from build123d import *

# Parameters (mm, degrees)
SKETCH1_W           = 60
SKETCH1_H           = 60
BOSS_EXTRUDE1_DEPTH = 1.2
FILLET1_R           = 4
SKETCH3_W           = 6.8
SKETCH3_H           = 20
BOSS_EXTRUDE3_DEPTH = 10
FILLET2_R           = 4
CUT_EXTRUDE1_DEPTH  = 100
CUT_EXTRUDE2_DEPTH  = 44.588989435
BOSS_EXTRUDE4_START = 10
BOSS_EXTRUDE4_DEPTH = 10
CUT_EXTRUDE4_REACH  = 55.014
SKETCH6_R           = 1.6
CUT_EXTRUDE5_REACH  = 62.463
SKETCH7_R           = 1.6
CUT_EXTRUDE6_REACH  = 62.463
SKETCH8_R           = 1.6
CUT_EXTRUDE7_REACH  = 62.463
SKETCH9_R           = 1.6
CUT_EXTRUDE8_REACH  = 62.463
SKETCH10_R          = 1.6


with BuildPart() as part:
    # Sketch1 → Boss-Extrude1 (new body)
    with BuildSketch(Plane(origin=(0, 0, 0), x_dir=(1, 0, 0), z_dir=(0, 1, 0))):
        Rectangle(SKETCH1_W, SKETCH1_H)
    extrude(amount=BOSS_EXTRUDE1_DEPTH)

    # Fillet1
    fillet1_edges = [part.edges().sort_by_distance(p)[0] for p in [
        (30, 0.6, 30),
        (-30, 0.6, 30),
        (-30, 0.6, -30),
        (30, 0.6, -30),
    ]]
    fillet(fillet1_edges, radius=FILLET1_R)

    # Sketch3 → Boss-Extrude3 (add)
    with BuildSketch(Plane(origin=(0, 1.2, 0), x_dir=(1, 0, 0), z_dir=(0, 1, 0))):
        with Locations((-25, 0)):
            Rectangle(SKETCH3_W, SKETCH3_H)
        with Locations((25, 0)):
            Rectangle(SKETCH3_W, SKETCH3_H)
    extrude(amount=BOSS_EXTRUDE3_DEPTH)

    # Fillet2
    fillet2_edges = [part.edges().sort_by_distance(p)[0] for p in [
        (-25, 11.2, -10),
        (-25, 11.2, 10),
        (25, 11.2, 10),
        (25, 11.2, -10),
    ]]
    fillet(fillet2_edges, radius=FILLET2_R)

    # Sketch4 → Cut-Extrude1 (cut)
    with BuildSketch(Plane.ZY.offset(28.4)):
        Polygon((0, 1.9), (0, 10.5), (-3.723909236, 8.35), (-3.723909236, 4.05), align=None)
        Polygon((3.723909236, 8.35), (0, 10.5), (0, 1.9), (3.723909236, 4.05), align=None)
    extrude(amount=-CUT_EXTRUDE1_DEPTH, mode=Mode.SUBTRACT)

    # Sketch5 → Cut-Extrude2 (cut, through all)
    with BuildSketch(Plane(origin=(0, 1.2, 0), x_dir=(1, 0, 0), z_dir=(0, 1, 0))):
        with BuildLine():
            Line((18.838235294, 1.694370386), (12.734380374, 8.316488925))
            ThreePointArc((12.734380374, 8.316488925), (10.731045286, 9.74540415), (8.322615669, 10.25))
            Line((8.322615669, 10.25), (-8.322615669, 10.25))
            ThreePointArc((-8.322615669, 10.25), (-10.731045286, 9.74540415), (-12.734380374, 8.316488925))
            Line((-12.734380374, 8.316488925), (-18.838235294, 1.694370386))
            ThreePointArc((-18.838235294, 1.694370386), (-19.5, 0), (-18.838235294, -1.694370386))
            Line((-18.838235294, -1.694370386), (-12.734380374, -8.316488925))
            ThreePointArc((-12.734380374, -8.316488925), (-10.731045286, -9.74540415), (-8.322615669, -10.25))
            Line((-8.322615669, -10.25), (8.322615669, -10.25))
            ThreePointArc((8.322615669, -10.25), (10.731045286, -9.74540415), (12.734380374, -8.316488925))
            Line((12.734380374, -8.316488925), (18.838235294, -1.694370386))
            ThreePointArc((18.838235294, -1.694370386), (19.5, 0), (18.838235294, 1.694370386))
        make_face()
    extrude(amount=-CUT_EXTRUDE2_DEPTH, mode=Mode.SUBTRACT)

    # Sketch5<3> → Boss-Extrude4 (add)
    with BuildSketch(Plane(origin=(0, 1.2, 0), x_dir=(1, 0, 0), z_dir=(0, 1, 0)).offset(BOSS_EXTRUDE4_START)):
        with BuildLine():
            Line((20.308823529, 3.049866694), (14.20496861, 9.671985234))
            ThreePointArc((14.20496861, 9.671985234), (11.533855159, 11.577205534), (8.322615669, 12.25))
            Line((8.322615669, 12.25), (-8.322615669, 12.25))
            ThreePointArc((-8.322615669, 12.25), (-11.533855159, 11.577205534), (-14.20496861, 9.671985234))
            Line((-14.20496861, 9.671985234), (-20.308823529, 3.049866694))
            ThreePointArc((-20.308823529, 3.049866694), (-21.5, 0), (-20.308823529, -3.049866694))
            Line((-20.308823529, -3.049866694), (-14.20496861, -9.671985234))
            ThreePointArc((-14.20496861, -9.671985234), (-11.533855159, -11.577205534), (-8.322615669, -12.25))
            Line((-8.322615669, -12.25), (8.322615669, -12.25))
            ThreePointArc((8.322615669, -12.25), (11.533855159, -11.577205534), (14.20496861, -9.671985234))
            Line((14.20496861, -9.671985234), (20.308823529, -3.049866694))
            ThreePointArc((20.308823529, -3.049866694), (21.5, 0), (20.308823529, 3.049866694))
        make_face()
        with BuildLine():
            Line((18.838235294, 1.694370386), (12.734380374, 8.316488925))
            ThreePointArc((12.734380374, 8.316488925), (10.731045286, 9.74540415), (8.322615669, 10.25))
            Line((8.322615669, 10.25), (-8.322615669, 10.25))
            ThreePointArc((-8.322615669, 10.25), (-10.731045286, 9.74540415), (-12.734380374, 8.316488925))
            Line((-12.734380374, 8.316488925), (-18.838235294, 1.694370386))
            ThreePointArc((-18.838235294, 1.694370386), (-19.5, 0), (-18.838235294, -1.694370386))
            Line((-18.838235294, -1.694370386), (-12.734380374, -8.316488925))
            ThreePointArc((-12.734380374, -8.316488925), (-10.731045286, -9.74540415), (-8.322615669, -10.25))
            Line((-8.322615669, -10.25), (8.322615669, -10.25))
            ThreePointArc((8.322615669, -10.25), (10.731045286, -9.74540415), (12.734380374, -8.316488925))
            Line((12.734380374, -8.316488925), (18.838235294, -1.694370386))
            ThreePointArc((18.838235294, -1.694370386), (19.5, 0), (18.838235294, 1.694370386))
        make_face(mode=Mode.SUBTRACT)
    extrude(amount=-BOSS_EXTRUDE4_DEPTH)

    # Cut-Extrude4: up to this face of the body (flat: up to its plane)
    cut_extrude4_end = Plane(part.part.faces().sort_by_distance((0, 6.2, -12.25))[0])
    # Sketch6 → Cut-Extrude4 (cut, up to the picked face)
    with BuildSketch(Plane.XY.offset(12.25), mode=Mode.PRIVATE) as cut_extrude4_sk1:
        with Locations((0, 6.2)):
            Circle(SKETCH6_R)
    cut_extrude4_tool1 = split(extrude(cut_extrude4_sk1.sketch, amount=-CUT_EXTRUDE4_REACH, mode=Mode.PRIVATE), bisect_by=cut_extrude4_end, keep=Keep.BOTH, mode=Mode.PRIVATE)
    add(cut_extrude4_tool1.solids().sort_by(Axis((0, 6.2, 12.25), (0, 0, -1)))[0], mode=Mode.SUBTRACT)

    # Sketch7 → Cut-Extrude5 (cut, up to next)
    with BuildSketch(Plane(origin=(-12.5, 0, 11.521718622), x_dir=(0.677748154223703, 0, 0.7352941176470567), z_dir=(-0.7352941176470567, 0, 0.677748154223703)), mode=Mode.PRIVATE) as cut_extrude5_sk1:
        with Locations((-7.018678015, 6.2)):
            Circle(SKETCH7_R)
    cut_extrude5_tool1 = extrude(cut_extrude5_sk1.sketch, amount=-CUT_EXTRUDE5_REACH, mode=Mode.PRIVATE) & part.part
    add(cut_extrude5_tool1.solids().sort_by_distance((-17.256896, 6.2, 6.360926))[0], mode=Mode.SUBTRACT)

    # Sketch8 → Cut-Extrude6 (cut, up to next)
    with BuildSketch(Plane(origin=(12.5, 0, 11.521718622), x_dir=(0.6777481542236974, 0, -0.735294117647062), z_dir=(0.735294117647062, 0, 0.6777481542236974)), mode=Mode.PRIVATE) as cut_extrude6_sk1:
        with Locations((7.018678015, 6.2)):
            Circle(SKETCH8_R)
    cut_extrude6_tool1 = extrude(cut_extrude6_sk1.sketch, amount=-CUT_EXTRUDE6_REACH, mode=Mode.PRIVATE) & part.part
    add(cut_extrude6_tool1.solids().sort_by_distance((17.256896, 6.2, 6.360926))[0], mode=Mode.SUBTRACT)

    # Sketch9 → Cut-Extrude7 (cut, up to next)
    with BuildSketch(Plane(origin=(-12.5, 0, -11.521718622), x_dir=(-0.6777481542236947, 0, 0.7352941176470644), z_dir=(-0.7352941176470644, 0, -0.6777481542236947)), mode=Mode.PRIVATE) as cut_extrude7_sk1:
        with Locations((7.018678015, 6.2)):
            Circle(SKETCH9_R)
    cut_extrude7_tool1 = extrude(cut_extrude7_sk1.sketch, amount=-CUT_EXTRUDE7_REACH, mode=Mode.PRIVATE) & part.part
    add(cut_extrude7_tool1.solids().sort_by_distance((-17.256896, 6.2, -6.360926))[0], mode=Mode.SUBTRACT)

    # Sketch10 → Cut-Extrude8 (cut, up to next)
    with BuildSketch(Plane(origin=(12.5, 0, -11.521718622), x_dir=(-0.6777481542237005, 0, -0.7352941176470591), z_dir=(0.7352941176470591, 0, -0.6777481542237005)), mode=Mode.PRIVATE) as cut_extrude8_sk1:
        with Locations((-7.018678015, 6.2)):
            Circle(SKETCH10_R)
    cut_extrude8_tool1 = extrude(cut_extrude8_sk1.sketch, amount=-CUT_EXTRUDE8_REACH, mode=Mode.PRIVATE) & part.part
    add(cut_extrude8_tool1.solids().sort_by_distance((17.256896, 6.2, -6.360926))[0], mode=Mode.SUBTRACT)


solid = part.part
Part model, mm, in its own coordinate system. A direction names the side the tool comes from. Give positions to 0.01 mm unless a question says otherwise; leave off trailing zeros. Loops run counter-clockwise (first coordinate to the right, second up) from the corner with the lowest first, then second, coordinate; pieces in that order, holes last. Notation, with made-up numbers: M 55,69.25 L 88,69.25 A11 cw 88,86.25 Z; hole C 63.5,38.25 d10. An arc over 180 degrees is marked long. Put each result on its own line as item: value. Start each with the question number.
1) Saw through at B-B (x = 0). List the corners of the cut face in (y, z).
2) Saw through at C-C (z = 13.5). List the corners of the cut face in (x, y).
3) Pull direction Z, two halves, no side cores. Call faces 5 (the cylindrical face through (-11.576, 6.27, 11.559)), 6 (the flat face through (2, 6, -12.25)), 7 (the cylindrical face through (-15.498, 6.681, 6.815)): +Z half, -Z half, draft (parallel to the pull), parting line (faces both ways), or undercut.
4) Saw through at D-D (y = 2.75). State how many separate pieces and enclosed holes the cut face has, then the cut area to 3 significant figures.
5) Probe probe 1 along Z at (x, y) = (3.5, 10); probe 2 along Z at (x, y) = (24, 4.5); probe 3 along Y at (x, z) = (0, -11). List the from-to ranges inside material, lowest first.
6) Flat gauge pins, fed straight in: pin 1 (5 mm diameter, centred on y = 7, z = 1, fed in from +X); pin 2 (3 mm diameter, centred on y = 7, z = -0.5, fed in from -X); pin 3 (1.5 mm diameter, centred on x = 22, y = 2, fed in from -Z). Where does each tip first touch, or does it go through?
7) Saw through at A-A (x = -23). List the corners of the cut face in (y, z), then the cut area to 3 significant figures.
8) 3-axis set-ups, long thin cutter, end or side, ignore diameter. For faces 1 (the flat face through (-28.4, 2.8, -2.1)), 2 (the cylindrical face through (-21.5, 6.3, 0)), 3 (the cylindrical face through (25.048, 9.997, 8.859)), 4 (the flat face through (-18.66, 6.27, 4.84)): which of +Z, -Z, +X, -X, +Y, -Y reach the whole face in a straight line?
Numbers:
1. outline: M 0,-30 L 1.2,-30 L 1.2,-12.25 L 4.6,-12.25 L 4.6,-10.25 L 0,-10.25 Z; M 0,10.25 L 4.6,10.25 L 4.6,12.25 L 1.2,12.25 L 1.2,30 L 0,30 Z; M 7.8,-12.25 L 11.2,-12.25 L 11.2,-10.25 L 7.8,-10.25 Z; M 7.8,10.25 L 11.2,10.25 L 11.2,12.25 L 7.8,12.25 Z
2. outline: M -30,0 L 30,0 L 30,1.2 L -30,1.2 Z
3. face 5: +Z half
3. face 6: -Z half
3. face 7: undercut
4. separate pieces: 5
4. enclosed holes: 1
4. area: 438 mm^2
5. probe 1: -12.25 to -10.25, 10.25 to 12.25
5. probe 2: -10 to -3.72, 3.72 to 10
5. probe 3: 0 to 4.6, 7.8 to 11.2
6. pin 1: x = 21.5
6. pin 2: x = -21.5
6. pin 3: z = -10
7. outline: M 0,-30 L 1.2,-30 L 1.2,-10 L 7.2,-10 A4 ccw 11.2,-6 L 11.2,6 A4 ccw 7.2,10 L 1.2,10 L 1.2,30 L 0,30 Z; hole M 1.9,0 L 4.05,-3.72 L 8.35,-3.72 L 10.5,0 L 8.35,3.72 L 4.05,3.72 Z
7. area: 217 mm^2
8. face 1: +Z, -Z, -X, +Y
8. face 2: +Y
8. face 3: +Z, +X, +Y
8. face 4: +Z, +Y
